Can you work these out from the model? Positions are in its coordinate system, mm. Face numbers are marked on the shaded views. A direction names the side the tool comes from. Give positions to 0.01 mm unless a question says otherwise; leave off trailing zeros. Order: outer loops, then holes, each group sorted by start corner. A loop starts at its lowest first (then second) coordinate and runs counter-clockwise, first axis right, second up. Notation, with made-up numbers: M 81,19.25 L 137,19.25 A24 cw 137,56.25 Z; hole C 79.25,51 d1. An arc over 180 degrees is marked long. Write each question's results on one line, items separated by ' | '.
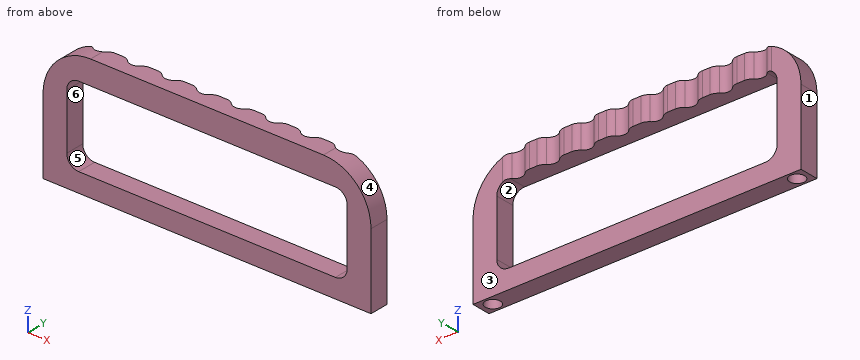
from build123d import *

# Parameters (mm, degrees)
BOSS_EXTRUDE1_DEPTH = 6.35
FILLET1_R           = 2.54
SKETCH1_3_W         = 6.35
SKETCH1_3_H         = 5.08
BOSS_EXTRUDE2_DEPTH = 26.289
SKETCH2_R           = 1.9939
CUT_EXTRUDE1_DEPTH  = 19.05
SKETCH3_W           = 5.08
SKETCH3_H           = 5.08
BOSS_EXTRUDE3_DEPTH = 74.91984
FILLET2_R           = 3.175
FILLET3_R           = 12.7


with BuildPart() as part:
    # Sketch1 → Boss-Extrude1 (new body)
    with BuildSketch(Plane.XY):
        with BuildLine():
            Line((-43.80992, 2.54), (-43.80992, -2.54))
            Line((-43.80992, -2.54), (43.80992, -2.54))
            Line((43.80992, -2.54), (43.80992, 2.54))
            Line((43.80992, 2.54), (34.572886058, 2.54))
            ThreePointArc((34.572886058, 2.54), (32.329618798, 1.016), (30.086351538, 2.54))
            Line((30.086351538, 2.54), (25.335852116, 2.54))
            ThreePointArc((25.335852116, 2.54), (23.092584856, 1.016), (20.849317595, 2.54))
            Line((20.849317595, 2.54), (16.098818173, 2.54))
            ThreePointArc((16.098818173, 2.54), (13.855550913, 1.016), (11.612283653, 2.54))
            Line((11.612283653, 2.54), (6.861784231, 2.54))
            ThreePointArc((6.861784231, 2.54), (4.618516971, 1.016), (2.375249711, 2.54))
            Line((2.375249711, 2.54), (-2.375249711, 2.54))
            ThreePointArc((-2.375249711, 2.54), (-4.618516971, 1.016), (-6.861784231, 2.54))
            Line((-6.861784231, 2.54), (-11.612283653, 2.54))
            ThreePointArc((-11.612283653, 2.54), (-13.855550913, 1.016), (-16.098818173, 2.54))
            Line((-16.098818173, 2.54), (-20.849317595, 2.54))
            ThreePointArc((-20.849317595, 2.54), (-23.092584856, 1.016), (-25.335852116, 2.54))
            Line((-25.335852116, 2.54), (-30.086351538, 2.54))
            ThreePointArc((-30.086351538, 2.54), (-32.329618798, 1.016), (-34.572886058, 2.54))
            Line((-34.572886058, 2.54), (-43.80992, 2.54))
        make_face()
    extrude(amount=BOSS_EXTRUDE1_DEPTH)

    # Fillet1
    fillet1_edges = [part.edges().sort_by_distance(p)[0] for p in [
        (-34.572886058, 2.54, 3.175),
        (-30.086351538, 2.54, 3.175),
        (-25.335852116, 2.54, 3.175),
        (-20.849317595, 2.54, 3.175),
        (-16.098818173, 2.54, 3.175),
        (-11.612283653, 2.54, 3.175),
        (-6.861784231, 2.54, 3.175),
        (-2.375249711, 2.54, 3.175),
        (2.375249711, 2.54, 3.175),
        (6.861784231, 2.54, 3.175),
        (11.612283653, 2.54, 3.175),
        (16.098818173, 2.54, 3.175),
        (20.849317595, 2.54, 3.175),
        (25.335852116, 2.54, 3.175),
        (30.086351538, 2.54, 3.175),
        (34.572886058, 2.54, 3.175),
    ]]
    fillet(fillet1_edges, radius=FILLET1_R)

    # Sketch1<3> → Boss-Extrude2 (add)
    with BuildSketch(Plane.XY):
        with Locations((-40.63492, 0)):
            Rectangle(SKETCH1_3_W, SKETCH1_3_H)
        Polygon((37.45992, 0), (37.45992, -2.54), (43.80992, -2.54), (43.80992, 2.54), (37.45992, 2.54), align=None)
    extrude(amount=-BOSS_EXTRUDE2_DEPTH)

    # Sketch2 → Cut-Extrude1 (cut)
    with BuildSketch(Plane(origin=(0, 0, -26.289), x_dir=(-1, 0, 0), z_dir=(0, 0, -1))):
        with Locations((-40.63492, 0)):
            Circle(SKETCH2_R)
        with Locations((40.63492, 0)):
            Circle(SKETCH2_R)
    extrude(amount=-CUT_EXTRUDE1_DEPTH, mode=Mode.SUBTRACT)

    # Sketch3 → Boss-Extrude3 (add)
    with BuildSketch(Plane.ZY.offset(-37.45992)):
        with Locations((-23.749, 0)):
            Rectangle(SKETCH3_W, SKETCH3_H)
    extrude(amount=BOSS_EXTRUDE3_DEPTH)

    # Fillet2
    fillet2_edges = [part.edges().sort_by_distance(p)[0] for p in [
        (37.45992, 0, -21.209),
        (-37.45992, 0, -21.209),
        (-37.45992, 0, 0),
        (37.45992, 0, 0),
    ]]
    fillet(fillet2_edges, radius=FILLET2_R)

    # Fillet3
    fillet3_edges = [part.edges().sort_by_distance(p)[0] for p in [
        (-43.80992, 0, 6.35),
        (43.80992, 0, 6.35),
    ]]
    fillet(fillet3_edges, radius=FILLET3_R)


solid = part.part
(1) Will these pins go through, and if not, where does the flat tip stop? P1, Ø4, axis at x = 33, z = 0, coming from the +Y side; P2, Ø2, axis at x = -40, y = 0.5, coming from the -Z side.
Data:
P1: stops at y = 2.37 | P2: stops at z = -7.24
(2) We'd pull the mould along Z, two halves only. Please class the marked faces 3, 4, 5 and 6: +Z half, -Z half, draft (parallel to the pull), parting line (faces both ways), or undercut.
Data:
face 3: draft | face 4: +Z half | face 5: undercut | face 6: undercut
(3) For the marked faces 1 and 2, which set-ups out of +Z, -Z, +X, -X, +Y, -Y let a thin tool reach every point of the face, with its end or its side?
Data:
face 1: +Z, -Z, -X, +Y, -Y | face 2: +Y, -Y
(4) I need wall thicknesses on L1, parallel to X at y = -2.3, z = -15; L2, parallel to Z at x = -9, y = -0.95; L3, parallel to X at y = 1.75, z = -9. Which ranges of each line are inside material? Lowest first, please. Write a range as from..to.
Data:
L1: x = -43.81..-37.46, 37.46..43.81 | L2: z = -26.29..-21.21, 0..6.35 | L3: x = -43.81..-41.59, -39.68..-37.46, 37.46..39.68, 41.59..43.81
(5) Imagine slicing it at A-A, the plane x = -28. Write out the boundary of the cut face in (y, z).
Data:
outline: M -2.54,-26.29 L 2.54,-26.29 L 2.54,-21.21 L -2.54,-21.21 Z; M -2.54,0 L 2.54,0 L 2.54,6.35 L -2.54,6.35 Z
(6) Imagine slicing it at D-D, the plane z = -5. Write out the boundary of the cut face in (x, y), plus the area to 3 significant figures.
Data:
outline: M -43.74,-2.54 L -37.46,-2.54 L -37.46,2.54 L -43.74,2.54 Z; M 37.46,-2.54 L 43.74,-2.54 L 43.74,2.54 L 37.46,2.54 Z | area: 63.8 mm2
(7) Imagine slicing it at C-C, the plane z = -19.5. Write out the boundary of the cut face in (x, y).
Data:
outline: M -43.81,-2.54 L -37.1,-2.54 L -37.1,2.54 L -43.81,2.54 Z; M 37.1,-2.54 L 43.81,-2.54 L 43.81,2.54 L 37.1,2.54 Z; hole C -40.63,0 d3.99; hole C 40.63,0 d3.99
(8) Imagine slicing it at B-B, the plane y = 0. Write out the boundary of the cut face in (x, z) (3 decimals), plus the area to 3 significant figures.
Data:
outline: M -43.81,-26.289 L -42.629,-26.289 L -42.629,-7.239 L -38.641,-7.239 L -38.641,-26.289 L 38.641,-26.289 L 38.641,-7.239 L 42.629,-7.239 L 42.629,-26.289 L 43.81,-26.289 L 43.81,-6.35 A12.7 ccw 31.11,6.35 L -31.11,6.35 A12.7 ccw -43.81,-6.35 Z; hole M -37.46,-18.034 A3.175 ccw -34.285,-21.209 L 34.285,-21.209 A3.175 ccw 37.46,-18.034 L 37.46,-3.175 A3.175 ccw 34.285,0 L -34.285,0 A3.175 ccw -37.46,-3.175 Z | area: 1,060 mm2
